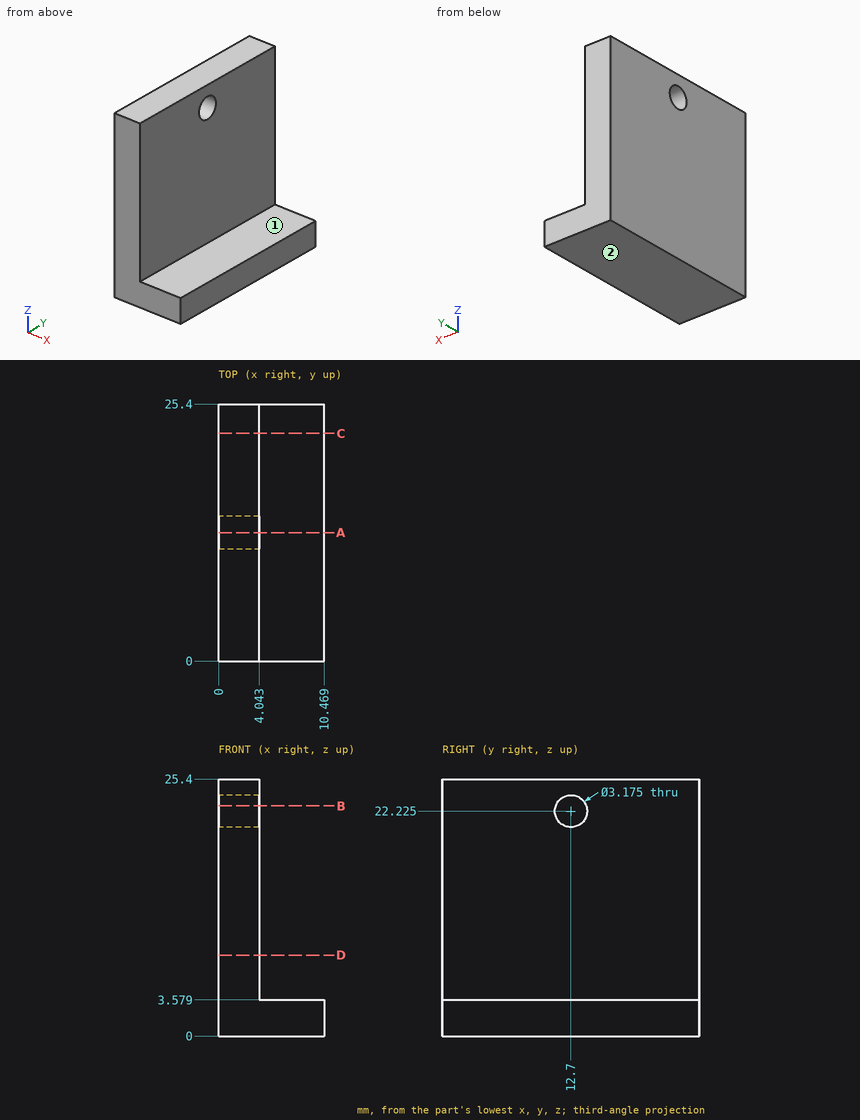
Drawing for the job (mm, zero at the part's lowest x, y, z). A direction names the side the tool comes from. Round coordinates to 2 decimals unless told otherwise and drop trailing zeros. Loops run counter-clockwise (first coordinate to the right, second up) from the corner with the lowest first, then second, coordinate; pieces in that order, holes last. Notation, with made-up numbers: (-39.75, 48.25) - (-7.75, 48.25) arc R20 ccw to (-7.75, 74.25) - close; hole circle Ø2 at (43.25, 32). An arc over 180 degrees is marked (long way). Write each question's results on one line, items separated by ' | '.
(1) Wall check: L1, parallel to Z at x = 2.7, y = 12.7; L2, parallel to X at y = 12.5, z = 16.25; L3, parallel to Z at x = 9.75, y = 19.5. Give the ranges that are in metal, low to high.
Answer below:
L1: z = 0 to 20.64, 23.81 to 25.4 | L2: x = 0 to 4.04 | L3: z = 0 to 3.58
(2) 3-axis set-ups, long thin cutter, end or side, ignore diameter. For the marked faces 1 and 2: which of +Z, -Z, +X, -X, +Y, -Y reach the whole face in a straight line?
Answer below:
face 1: +Z, +X, +Y, -Y | face 2: -Z, +X, -X, +Y, -Y
(3) Saw through at C-C, the plane y = 22.5. List the corners of the cut face in (x, z).
Answer below:
outline: (0, 0) - (10.47, 0) - (10.47, 3.58) - (4.04, 3.58) - (4.04, 25.4) - (0, 25.4) - close
(4) Saw through at D-D, the plane z = 8. List the corners of the cut face in (x, y).
Answer below:
outline: (0, 0) - (4.04, 0) - (4.04, 25.4) - (0, 25.4) - close
(5) Saw through at A-A, the plane y = 12.7. List the corners of the cut face in (x, z), then the cut area to 3 significant figures.
Answer below:
outline: (0, 0) - (10.47, 0) - (10.47, 3.58) - (4.04, 3.58) - (4.04, 20.64) - (0, 20.64) - close; (0, 23.81) - (4.04, 23.81) - (4.04, 25.4) - (0, 25.4) - close | area: 113 mm^2
(6) Pin check, flat tips, straight feed: pin 1 (3 mm diameter, centred on x = 6.5, y = 8.5, fed in from +Z); pin 2 (5 mm diameter, centred on x = 7.5, z = 8.5, fed in from +Y); pin 3 (11 mm diameter, centred on y = 14.5, z = 15, fed in from +X). Stop position of each tip, or through.
Answer below:
pin 1: stops at z = 3.58 | pin 2: passes through | pin 3: stops at x = 4.04
(7) Saw through at B-B, the plane z = 22.75. List the corners of the cut face in (x, y).
Answer below:
outline: (0, 0) - (4.04, 0) - (4.04, 11.2) - (0, 11.2) - close; (0, 14.2) - (4.04, 14.2) - (4.04, 25.4) - (0, 25.4) - close
